from build123d import *

# Parameters (mm, degrees)
SKETCH_1_R               = 40
EXTRUDE_1_DEPTH          = 10
SKETCH_2_R               = 11
EXTRUDE_2_DEPTH          = 8
SKETCH_3_R               = 3
CUT_EXTRUDE_1_DEPTH      = 60.363288319
M4X0_7_1_REACH           = 68.31
M4X0_7_1_BORE_R          = 1.65
CUT_EXTRUDE_2_DEPTH      = 1
CUT_EXTRUDE_2_DEPTH_BACK = 1
SKETCH_5_OUTSIDE_W       = 104.912
SKETCH_5_OUTSIDE_H       = 104.912
SKETCH_5_OUTSIDE_R       = 38


with BuildPart() as part:
    # ｽｹｯﾁ1 → ﾎﾞｽ - 押し出し1 (new body)
    with BuildSketch(Plane.XY):
        Circle(SKETCH_1_R)
    extrude(amount=EXTRUDE_1_DEPTH)

    # ｽｹｯﾁ2 → ﾎﾞｽ - 押し出し2 (add)
    with BuildSketch(Plane.XY.offset(10)):
        Circle(SKETCH_2_R)
    extrude(amount=EXTRUDE_2_DEPTH)

    # ｽｹｯﾁ3 → ｶｯﾄ - 押し出し1 (cut, through all)
    with BuildSketch(Plane.XY.offset(18)):
        Circle(SKETCH_3_R)
    extrude(amount=-CUT_EXTRUDE_1_DEPTH, mode=Mode.SUBTRACT)

    # M4x0.7 ねじ穴1 bore (on position points) → M4x0.7 ねじ穴1 (cut, up to next)
    with BuildSketch(Plane(origin=(0, -11, 14), x_dir=(-1, 0, 0), z_dir=(0, -1, 0)), mode=Mode.PRIVATE) as m4x0_7_1_sk1:
        Circle(M4X0_7_1_BORE_R)
    m4x0_7_1_tool1 = extrude(m4x0_7_1_sk1.sketch, amount=-M4X0_7_1_REACH, mode=Mode.PRIVATE) & part.part
    add(m4x0_7_1_tool1.solids().sort_by_distance((0, -11, 14))[0], mode=Mode.SUBTRACT)

    # ｽｹｯﾁ5 outside → ｶｯﾄ - 押し出し2 (cut, two sides: drawn at the far end of the back side and taken through both)
    with BuildSketch(Plane(origin=(0, 0, 5), x_dir=(-1, 0, 0), z_dir=(0, 0, -1)).offset(-CUT_EXTRUDE_2_DEPTH_BACK)):
        Rectangle(SKETCH_5_OUTSIDE_W, SKETCH_5_OUTSIDE_H)
        Circle(SKETCH_5_OUTSIDE_R, mode=Mode.SUBTRACT)
    extrude(amount=CUT_EXTRUDE_2_DEPTH + CUT_EXTRUDE_2_DEPTH_BACK, mode=Mode.SUBTRACT)


solid = part.part
Design review of the part built by this model. Coordinates are the model's own, in mm. A direction names the side the tool comes from. Coordinates: 2 decimals unless noted, no trailing zeros. Order: outer loops, then holes, each group sorted by start corner. A loop starts at its lowest first (then second) coordinate and runs counter-clockwise, first axis right, second up.
Item 1: Take a section at C-C, the plane z = 2.5. Write out the cut boundary in (x, y).
Item 2: For pin 1 Ø6 at (x, y) = (-24, -31.5) entering from +Z; pin 2 Ø8 at (x, z) = (21, 12.5) entering from -Y; pin 3 Ø6 at (x, z) = (-11.5, 10) entering from +Y, all flat-tipped, find the tip position at first contact; note any pin that passes through.
Item 3: Take a section at B-B, the plane y = 0. Write out the cut boundary in (x, z), then the cut area to 3 significant figures.
Item 4: Take a section at D-D, the plane y = 26. Write out the cut boundary in (x, z), then the cut area to 3 significant figures.
Item 5: For faces 4 (the cylindrical face through (-8.67, -39.05, 7.97)), 5 (the flat face through (-35.4, -14.6, 4)), 6 (the flat face through (8, -8, 10)), list the 3-axis set-ups (+Z, -Z, +X, -X, +Y, -Y) from which the entire face can be reached by the end or side of a thin tool; tool diameter is ignored.
Item 6: For line 1 (Z direction, x = 0, y = -7); line 2 (Y direction, x = 0, z = 4.25); line 3 (Y direction, x = 0, z = 7.5), list the stretches that pass through material, from the lowest coordinate up.
Item 7: Take a section at A-A, the plane x = 0. Write out the cut boundary in (y, z).
Item 8: The part is to be moulded in two halves that separate along Y. For faces 1 (the cylindrical face through (0.215, -6.812, 12.364)), 2 (the cylindrical face through (0, 3, 9)), 3 (the cylindrical face through (-8.67, -39.05, 1.97)), say which applies: pulls with the +Y half, pulls with the -Y half, needs draft (parallel to the pull), parting line crosses it, or undercut.
The answers:
1. outline: circle Ø80 at (0, 0); hole circle Ø6 at (0, 0)
2. pin 1: stops at z = 10
2. pin 2: stops at y = -35.78
2. pin 3: stops at y = 39.09
3. outline: (-40, 0) - (-3, 0) - (-3, 18) - (-11, 18) - (-11, 10) - (-40, 10) - (-40, 6) - (-38, 6) - (-38, 4) - (-40, 4) - close; (3, 0) - (40, 0) - (40, 4) - (38, 4) - (38, 6) - (40, 6) - (40, 10) - (11, 10) - (11, 18) - (3, 18) - close
3. area: 860 mm2
4. outline: (-30.4, 0) - (30.4, 0) - (30.4, 4) - (27.71, 4) - (27.71, 6) - (30.4, 6) - (30.4, 10) - (-30.4, 10) - (-30.4, 6) - (-27.71, 6) - (-27.71, 4) - (-30.4, 4) - close
4. area: 597 mm2
5. face 4: +Z, -Z
5. face 5: none
5. face 6: +Z
6. line 1: z = 0 to 12.35, 15.65 to 18
6. line 2: y = -38 to -3, 3 to 38
6. line 3: y = -40 to -3, 3 to 40
7. outline: (-40, 0) - (-3, 0) - (-3, 12.35) - (-11, 12.35) - (-11, 10) - (-40, 10) - (-40, 6) - (-38, 6) - (-38, 4) - (-40, 4) - close; (-11, 15.65) - (-3, 15.65) - (-3, 18) - (-11, 18) - close; (3, 0) - (40, 0) - (40, 4) - (38, 4) - (38, 6) - (40, 6) - (40, 10) - (11, 10) - (11, 18) - (3, 18) - close
8. face 1: needs draft
8. face 2: undercut
8. face 3: parting line crosses it
